Verification items for the finished model (mm, model axes). Coordinates: 2 decimals unless noted, no trailing zeros. Loops run counter-clockwise (first coordinate to the right, second up) from the corner with the lowest first, then second, coordinate; pieces in that order, holes last.
Q1. Material ranges on probe 1 along Y at (x, z) = (19, 0.6); probe 2 along X at (y, z) = (25.5, 0.8); probe 3 along Y at (x, z) = (20, 1.3), recorded low to high.
Q2. Sectioned sample at C-C (z = 1). Count the separate pieces of the cut face and the enclosed holes in it, then the cut area to 3 significant figures.
Q3. Sectioned sample at B-B (y = -25.5). Enter the section's corners in (x, z), then the cut area to 3 significant figures.
Q4. Go/stop test with a flat-tipped pin: P1, Ø4, axis at x = 0, y = 8.18, coming from the -Z side. Record where the tip stops, or that it passes through.
Q5. Mould release check, pull along Y, two halves, no side actions. Record for faces 1 (the face through (19.371, -9.564, 0.751)), 2 (the face through (14.451, -21.906, 0.751)), 3 (the face through (-34.036, 5, 1)), 4 (the face through (29.653, -25.262, 0.773)): +Y half, -Y half, draft (parallel to the pull), parting line (faces both ways), or undercut.
Q6. Sectioned sample at A-A (x = 0). Enter the section's corners in (y, z).
Autodesk Inventor part; units mm, degrees
ref_plane "YZ Plane" through (0, 0, 0) normal (1, 0, 0) x (0, 1, 0)
ref_plane "XZ Plane" through (0, 0, 0) normal (0, 1, 0) x (-1, 0, 0)
ref_plane "XY Plane" through (0, 0, 0) normal (0, 0, 1) x (1, 0, 0)
sketch "Sketch1" plane through (0, 0, 0) normal (0, 0, 1) x (1, 0, 0)
  line L0 (-34.036, -29.7688) -> (34.036, -29.7688)
  line L1 (34.036, -29.7688) -> (34.036, 29.7688)
  line L2 (34.036, 29.7688) -> (-34.036, 29.7688)
  line L3 (-34.036, 29.7688) -> (-34.036, -29.7688)
  line L4 (-34.036, -29.7688) -> (34.036, 29.7688) construction
  line L5 (34.036, -29.7688) -> (-34.036, 29.7688) construction
  point P0 (0, 0)
  dimension "d0" = 68.072
  dimension "d1" = 59.5376
extrude "Extrusion1" add sketch "Sketch1" along normal blind 1.524
sketch "Sketch2" plane through (0, 0, 1.524) normal (0, 0, 1) x (1, 0, 0)
  line L0 (34.036, 29.7688) -> (-34.036, 29.7688)
  line L1 (-34.036, -29.7688) -> (34.036, -29.7688)
  line L2 (-34.036, 29.7688) -> (-34.036, -29.7688)
  line L3 (34.036, -29.7688) -> (34.036, 29.7688)
  point P0 (0, 0)
  point P1 (-18.796, 8.1788)
  point P2 (-18.796, -8.1788)
  point P3 (0, 8.1788)
  point P4 (0, -8.1788)
  point P5 (18.796, 8.1788)
  point P6 (18.796, -8.1788)
  dimension "d4" = 21.59
  dimension "d5" = 21.59
  dimension "d6" = 15.24
  dimension "d7" = 15.24
  dimension "d8" = 37.592
  dimension "d9" = 18.796
hole "Hole1" at (-18.796, 8.1788, 1.524) at (-18.796, -8.1788, 1.524) at (0, 8.1788, 1.524) at (0, -8.1788, 1.524) at (18.796, 8.1788, 1.524) at (18.796, -8.1788, 1.524) direction (0, 0, -1) diameter 3 depth 25.4 tip angle 118
chamfer "Chamfer1" distance 8.89 angle 45 2 edges at (-34.036, -29.7688, 0.762) (34.036, -29.7688, 0.762)
sketch "Sketch4" plane through (0, 0, 1.524) normal (0, 0, 1) x (1, 0, 0)
  circle A0 centre (-14.605, 25.3976) radius 3.1496
  circle A1 centre (14.605, 25.3976) radius 3.1496
  circle A2 centre (-14.605, -25.4024) radius 3.1496
  circle A3 centre (14.605, -25.4024) radius 3.1496
  point P0 (0, 0)
hole "Hole3" at (-14.605, 25.3976, 1.524) at (14.605, 25.3976, 1.524) at (14.605, -25.4024, 1.524) at (-14.605, -25.4024, 1.524) direction (0, 0, -1) diameter 7 end through all
properties part number "DPLX_P030_VIPE Insulation Bottom" material "Polyethylene, High Density"
Geometry check:
1. probe 1: y = -29.77 to -9.66, -6.69 to 6.69, 9.66 to 29.77
1. probe 2: x = -34.04 to -18.1, -11.11 to 11.11, 18.1 to 34.04
1. probe 3: y = -29.77 to -9.07, -7.28 to 7.28, 9.07 to 29.77
2. separate pieces: 1
2. enclosed holes: 10
2. area: 3,780 mm2
3. outline: (-29.41, 0) - (-18.1, 0) - (-18.1, 1.52) - (-29.41, 1.52) - close; (-11.11, 0) - (11.11, 0) - (11.11, 1.52) - (-11.11, 1.52) - close; (18.1, 0) - (29.41, 0) - (29.41, 1.52) - (18.1, 1.52) - close
3. area: 68.3 mm2
4. P1: stops at z = 0
5. face 1: undercut
5. face 2: undercut
5. face 3: draft
5. face 4: -Y half
6. outline: (-29.77, 0) - (-9.68, 0) - (-9.68, 1.52) - (-29.77, 1.52) - close; (-6.68, 0) - (6.68, 0) - (6.68, 1.52) - (-6.68, 1.52) - close; (9.68, 0) - (29.77, 0) - (29.77, 1.52) - (9.68, 1.52) - close
